Autodesk Inventor part; units mm, degrees
ref_plane "YZ Plane" through (0, 0, 0) normal (1, 0, 0) x (0, 1, 0)
ref_plane "XZ Plane" through (0, 0, 0) normal (0, 1, 0) x (-1, 0, 0)
ref_plane "XY Plane" through (0, 0, 0) normal (0, 0, 1) x (1, 0, 0)
sketch "Sketch1" plane through (0, 0, 0) normal (0, 1, 0) x (-1, 0, 0)
  line L0 (0, 0) -> (-590, 0)
  line L1 (-590, 0) -> (-590, -165.9671)
  line L2 (-590, -165.9671) -> (0, -165.9671)
  line L3 (0, -165.9671) -> (0, 0)
  line L4 (0, -165.9671) -> (0, -270)
  line L5 (0, -270) -> (-590, -165.9671)
  dimension "d0" = 590
  dimension "d28" = 270
  dimension "d29" = 10
extrude "Extrusion1" add sketch "Sketch1" along normal blind 3
sketch "Sketch3" plane through (0, 3, 0) normal (0, 1, 0) x (1, 0, 0)
  circle A0 centre (585.75, 41.75) radius 1.25
  circle A1 centre (585.75, 78.75) radius 1.25
  line L0 (590, 0) -> (590, 165.9671)
  line L1 (0, 0) -> (590, 0)
  dimension "d15" = 2.5
  dimension "d16" = 4.25
  dimension "d17" = 4.25
  dimension "d18" = 2.5
  dimension "d19" = 41.75
  dimension "d20" = 37
extrude "Extrusion3" cut sketch "Sketch3" along normal through all both and the other way through all
sketch "Sketch4" plane through (0, 3, 0) normal (0, 1, 0) x (1, 0, 0)
  circle A0 centre (490, 60) radius 12
  line L0 (0, 0) -> (590, 0)
  line L1 (590, 0) -> (590, 165.9671)
  line L2 (14.1705, 156) -> (20.1705, 156)
  line L3 (20.1705, 156) -> (20.1705, 144)
  line L4 (20.1705, 144) -> (14.1705, 144)
  line L5 (14.1705, 144) -> (14.1705, 156)
  line L6 (15, 114) -> (21, 114)
  line L7 (21, 114) -> (21, 102)
  line L8 (21, 102) -> (15, 102)
  line L9 (15, 102) -> (15, 114)
  line L10 (15, 72) -> (21, 72)
  line L11 (21, 72) -> (21, 60)
  line L12 (21, 60) -> (15, 60)
  line L13 (15, 60) -> (15, 72)
  circle A1 centre (17.1705, 176) radius 1.25
  circle A2 centre (18, 40) radius 1.25
  line L14 (18, 60) -> (18, 40) construction
  dimension "d23" = 24
  dimension "d24" = 60
  dimension "d25" = 100
  dimension "d30" = 6
  dimension "d31" = 12
  dimension "d32" = 30
  dimension "d33" = 30
  dimension "d34" = 2.5
  dimension "d35" = 2.5
  dimension "d36" = 20
  dimension "d37" = 20
  dimension "d38" = 60
extrude "Extrusion4" cut sketch "Sketch4" against normal through all contours A0 | A1 | A2
equation "\"d16\" = d17"
equation "\"d18\" = d15"
equation "\"d33\" = d32"
equation "\"d34\" = d35"
equation "\"d37\" = d36"
properties part number "pinball-case-left-wall-outer"
Read the model definition and answer for the solid it produces. Units are mm, in the model's axes. Coordinates: 2 decimals unless noted, no trailing zeros. Order: outer loops, then holes, each group sorted by start corner. A loop starts at its lowest first (then second) coordinate and runs counter-clockwise, first axis right, second up. Notation, with made-up numbers: (-17.5, 31) - (14.5, 31) arc R11 cw to (14.5, 50) - close; hole circle Ø8 at (77.5, 14). An arc over 180 degrees is marked (long way). Use one line per item in the form item = value.
(1) Section B-B, the plane x = 490 is taken. Give the vertices of the cut face in (y, z).
Computed values:
outline = (0, -183.6) - (3, -183.6) - (3, -72) - (0, -72) - close; (0, -48) - (3, -48) - (3, 0) - (0, 0) - close
(2) Section D-D, the plane x = 62 is taken. Give the vertices of the cut face in (y, z).
Computed values:
outline = (0, -259.07) - (3, -259.07) - (3, 0) - (0, 0) - close
(3) For a pull along X with two mould halves and no side action, classify faces 1 (the face through (299, 0, -103)), 2 (the face through (501.085, 1.521, -55.404)), 3 (the face through (290.87, 1.48, -218.71)) as pulls with the +X half, pulls with the -X half, needs draft (parallel to the pull), parting line crosses it, or undercut.
Computed values:
face_1 = needs draft
face_2 = undercut
face_3 = pulls with the +X half
(4) Section A-A, the plane y = 2 is taken. Give the vertices of the cut face in (x, z), then the cut area to 3 significant figures.
Computed values:
outline = (0, -270) - (590, -165.97) - (590, 0) - (0, 0) - close; hole circle Ø2.5 at (17.17, -176); hole circle Ø2.5 at (18, -40); hole circle Ø24 at (490, -60); hole circle Ø2.5 at (585.75, -78.75); hole circle Ø2.5 at (585.75, -41.75)
area = 128,000 mm²
(5) Section C-C, the plane z = -211 is taken. Give the vertices of the cut face in (x, y), then the cut area to 3 significant figures.
Computed values:
outline = (0, 0) - (334.61, 0) - (334.61, 3) - (0, 3) - close
area = 1,000 mm²
(6) Straight lines are drawn through the part: L1, parallel to X at y = 1.1, z = -60; L2, parallel to X at y = 2.25, z = -78.75; L3, parallel to Z at x = 490, y = 0.85. For each, find the intervals that lie inside material, in ascending order.
Computed values:
L1 = 0 to 478, 502 to 590
L2 = 0 to 584.5, 587 to 590
L3 = -183.6 to -72, -48 to 0
